Input: part model. Units: mm. Frame: model coordinates. Coordinates: 2 decimals unless noted, no trailing zeros. Order: outer loops, then holes, each group sorted by start corner. A loop starts at its lowest first (then second) coordinate and runs counter-clockwise, first axis right, second up.
from build123d import *

# Parameters (mm, degrees)
SKETCH1_R           = 10
BOSS_EXTRUDE1_DEPTH = 161.1


with BuildPart() as part:
    # Sketch1 → Boss-Extrude1 (new body, symmetric)
    with BuildSketch(Plane(origin=(0, 0, 0), x_dir=(1, 0, 0), z_dir=(0, 1, 0))):
        Circle(SKETCH1_R)
    extrude(amount=BOSS_EXTRUDE1_DEPTH, both=True)

    # Sketch3 → M5x0.8 Tapped Hole1 (revolve, cut)
    with BuildSketch(Plane(origin=(0, 161.1, 0), x_dir=(0, 0, 1), z_dir=(1, 0, 0))):
        Polygon((0, 0), (0, 23.7618073), (2.1, 22.5), (2.1, 0), align=None)
    m5x0_8_tapped_hole1 = revolve(axis=Axis((0, 167.45, 0), (0, -1, 0)), mode=Mode.SUBTRACT)

    # Mirror1: M5x0.8 Tapped Hole1 across plane
    add(m5x0_8_tapped_hole1.mirror(Plane.ZX), mode=Mode.SUBTRACT)


solid = part.part
Item 1: Ray query, probe 1 along Z at (x, y) = (0, 147.75); probe 2 along X at (y, z) = (127.5, -0.5); probe 3 along X at (y, z) = (-135.5, -1). Return the intervals inside material, ascending.
Response values:
probe 1: z = -10 to -2.1, 2.1 to 10
probe 2: x = -9.99 to 9.99
probe 3: x = -9.95 to 9.95
Item 2: Cut plane B-B on x = 7.25. Return loops of the section in (y, z), then the cut area to 3 significant figures.
Response values:
outline: (-161.1, -6.89) - (161.1, -6.89) - (161.1, 6.89) - (-161.1, 6.89) - close
area: 4,440 mm2
Item 3: Pin query (flat end, axial travel): pin 1 Ø4 at (y, z) = (42, -7) entering from +X; pin 2 Ø6 at (x, y) = (6.5, 123.5) entering from -Z; pin 3 Ø10 at (y, z) = (-19, -5) entering from +X; pin 4 Ø3 at (y, z) = (94, 4.5) entering from +X. Return the tip coordinate at first contact, or that it passes through.
Response values:
pin 1: stops at x = 8.66
pin 2: stops at z = -9.37
pin 3: stops at x = 10
pin 4: stops at x = 9.54
Item 4: Cut plane C-C on z = 5.75. Return loops of the section in (x, y), then the cut area to 3 significant figures.
Response values:
outline: (-8.18, -161.1) - (8.18, -161.1) - (8.18, 161.1) - (-8.18, 161.1) - close
area: 5,270 mm2
Item 5: Cut plane A-A on y = 81. Return loops of the section in (x, z).
Response values:
outline: circle Ø20 at (0, 0)
